Autodesk Inventor part; units mm, degrees
ref_plane "YZ Plane" through (0, 0, 0) normal (1, 0, 0) x (0, 1, 0)
ref_plane "XZ Plane" through (0, 0, 0) normal (0, 1, 0) x (-1, 0, 0)
ref_plane "XY Plane" through (0, 0, 0) normal (0, 0, 1) x (1, 0, 0)
sketch "Sketch1" plane through (0, 0, 0) normal (0, 0, 1) x (1, 0, 0)
  circle A0 centre (0, 0) radius 10
  dimension "d0" = 20
extrude "Extrusion1" add sketch "Sketch1" along normal blind 2
sketch "Sketch2" plane through (0, 0, 0) normal (0, 0, -1) x (-1, 0, 0)
  circle A0 centre (0, 0) radius 5.5
  circle A1 centre (0, 0) radius 3.55
  dimension "d3" = 11
  dimension "d6" = 7.1
extrude "Extrusion2" add sketch "Sketch2" against normal blind 30 contours A0 | A1
sketch "Sketch3" plane through (0, 0, 0) normal (0, 0, -1) x (-1, 0, 0)
  point P0 (0, 0)
sketch "Sketch4" plane through (0, 0, 0) normal (0, 0, -1) x (-1, 0, 0)
  point P0 (0, 0)
sketch "Sketch5" plane through (0, 0, 0) normal (0, 0, -1) x (-1, 0, 0)
  circle A0 centre (0, 0) radius 4
  dimension "d7" = 8
extrude "Extrusion3" cut sketch "Sketch5" against normal blind 30
sketch "Sketch6" plane through (0, 0, 2) normal (0, 0, 1) x (1, 0, 0)
  circle A0 centre (7, 2) radius 1
  circle A1 centre (7, -2) radius 1
  circle A2 centre (-7, 2) radius 1
  circle A3 centre (-7, -2) radius 1
  point P0 (0, 0)
  dimension "d16" = 2
  dimension "d17" = 7
  dimension "d18" = 2
  dimension "d19" = 2
  dimension "d20" = 7
  dimension "d21" = 2
  dimension "d53" = 2
  dimension "d54" = 7
  dimension "d55" = 2
  dimension "d56" = 2
  dimension "d57" = 7
  dimension "d58" = 2
extrude "Extrusion4" cut sketch "Sketch6" against normal blind 2
sketch "Sketch7" plane through (0, 0, 0) normal (0, 0, -1) x (-1, 0, 0)
  point P0 (0, 0)
sketch "Sketch8" plane through (0, 0, 0) normal (0, 0, -1) x (-1, 0, 0)
  circle A0 centre (-29.1938, 0) radius 12
  point P0 (0, 0)
  dimension "d24" = 24
extrude "Extrusion5" add sketch "Sketch8" against normal blind 2
sketch "Sketch9" plane through (29.1938, 0, 0) normal (0, 0, -1) x (-1, 0, 0)
  circle A0 centre (0, 0) radius 6
  point P0 (29.1938, 0)
  dimension "d27" = 12
extrude "Extrusion6" cut sketch "Sketch9" against normal blind 1
sketch "Sketch10" plane through (29.1938, 0, 0) normal (0, 0, -1) x (-1, 0, 0)
  point P0 (29.1938, 0)
  point P1 (0, 0)
sketch "Sketch11" plane through (29.1938, 0, 0) normal (0, 0, -1) x (-1, 0, 0)
  circle A0 centre (7.6938, 2) radius 1
  circle A1 centre (-8.3062, 2) radius 1
  circle A2 centre (-8.3062, -2) radius 1
  circle A3 centre (7.6938, -2) radius 1
  point P0 (29.1938, 0)
  dimension "d30" = 21.5
  dimension "d31" = 2
  dimension "d32" = 16
  dimension "d33" = 2
  dimension "d34" = 2
  dimension "d35" = 0
  dimension "d36" = 0
  dimension "d37" = 4
  dimension "d38" = 2
  dimension "d40" = 2
  dimension "d41" = 4
extrude "Extrusion7" cut sketch "Sketch11" against normal blind 2
sketch "Sketch12" plane through (29.1938, 0, 2) normal (0, 0, 1) x (1, 0, 0)
  circle A0 centre (0, 0) radius 4.55
  point P0 (-29.1938, 0)
  dimension "d44" = 9.1
extrude "Extrusion8" cut sketch "Sketch12" against normal blind 1
sketch "Sketch13" plane through (29.1938, 0, 0) normal (0, 0, -1) x (-1, 0, 0)
  line L0 (19.6938, 1) -> (11.6938, 1)
  line L1 (11.6938, 1) -> (11.6938, -1)
  line L2 (11.6938, -1) -> (19.6938, -1)
  line L3 (19.6938, -1) -> (19.6938, 1)
  point P0 (29.1938, 0)
  dimension "d47" = 8
  dimension "d48" = 2
  dimension "d49" = 1
  dimension "d50" = 9.5
extrude "Extrusion9" add sketch "Sketch13" against normal blind 1
sketch "Sketch14" plane through (29.1938, 0, 2) normal (0, 0, 1) x (1, 0, 0)
  point P0 (-29.1938, 0)
sketch "Sketch15" plane through (29.1938, 0, 2) normal (0, 0, 1) x (1, 0, 0)
  circle A0 centre (0, 0) radius 12
  point P0 (-29.1938, 0)
  dimension "d59" = 24
extrude "Extrusion10" add sketch "Sketch15" along normal blind 22
sketch "Sketch16" plane through (29.1938, 0, 24) normal (0, 0, 1) x (1, 0, 0)
  circle A0 centre (0, 0) radius 10.5
  point P0 (-29.1938, 0)
  dimension "d62" = 21
extrude "Extrusion11" cut sketch "Sketch16" against normal blind 23
properties part number "Bobbin01"
Could you check a few things on this model? Use its own coordinates, in mm. A direction names the side the tool comes from. Give positions to 0.01 mm unless a question says otherwise; leave off trailing zeros. Order: outer loops, then holes, each group sorted by start corner. A loop starts at its lowest first (then second) coordinate and runs counter-clockwise, first axis right, second up.
1. Suppose I cut it at A-A (x = 0). Write out the boundary of the cut face in (y, z).
Answers below:
outline: (-10, 0) - (-4, 0) - (-4, 30) - (-5.5, 30) - (-5.5, 2) - (-10, 2) - close; (4, 0) - (10, 0) - (10, 2) - (5.5, 2) - (5.5, 30) - (4, 30) - close
2. Suppose I cut it at B-B (y = 0). Write out the boundary of the cut face in (x, z), plus the area to 3 significant figures.
Answers below:
outline: (-10, 0) - (-4, 0) - (-4, 30) - (-5.5, 30) - (-5.5, 2) - (-10, 2) - close; (4, 0) - (23.19, 0) - (23.19, 1) - (18.69, 1) - (18.69, 24) - (17.19, 24) - (17.19, 1) - (10, 1) - (10, 2) - (5.5, 2) - (5.5, 30) - (4, 30) - close; (35.19, 0) - (41.19, 0) - (41.19, 24) - (39.69, 24) - (39.69, 1) - (35.19, 1) - close
area: 196 mm2
3. Thinking about a two-plate mould opening in Y: for faces 1 (the cylindrical face through (20.576, 1.617, 0.493)), 2 (the cylindrical face through (6.2, 1.4, 1)), 3 (the flat face through (15, 0, 0)), 4 (the flat face through (13.5, 1, 0.5)), which applies, +Y half, -Y half, draft (parallel to the pull), parting line (faces both ways), or undercut?
Answers below:
face 1: undercut
face 2: undercut
face 3: draft
face 4: +Y half
4. Suppose I cut it at D-D (x = 21.5). Write out the boundary of the cut face in (y, z).
Answers below:
outline: (-9.21, 0) - (-3, 0) - (-3, 1) - (-7.15, 1) - (-7.15, 24) - (-9.21, 24) - close; (-1, 0) - (1, 0) - (1, 1) - (-1, 1) - close; (3, 0) - (9.21, 0) - (9.21, 24) - (7.15, 24) - (7.15, 1) - (3, 1) - close
5. For pin 1 (1.5 mm diameter, centred on y = 1.5, z = 9, fed in from -X); pin 2 (6 mm diameter, centred on x = 33, z = 11, fed in from -Y); pin 3 (12 mm diameter, centred on x = 27.5, y = -5.5, fed in from +Z), each with a flat end and sliding along its axis, tell me the tip position at first contact or that it passes through.
Answers below:
pin 1: stops at x = -5.45
pin 2: stops at y = -11.97
pin 3: stops at z = 24
6. Which directions (+Z, -Z, +X, -X, +Y, -Y) give clear straight access to the entire face, cutting with the end or side of a thin tool? Please do faces 5 (the flat face through (4, -4, 2)), 6 (the flat face through (29, -11, 24)), 7 (the flat face through (14, 0, 1)).
Answers below:
face 5: +Z
face 6: +Z, +X, +Y, -Y
face 7: +Z, +Y, -Y
7. I need wall thicknesses on L1, parallel to Y at x = -7, z = 0.9; L2, parallel to Y at x = 0, z = 25.5; L3, parallel to Y at x = 29, z = 20.25. Which ranges of each line are inside material? Lowest first, please.
Answers below:
L1: y = -7.14 to -3, -1 to 1, 3 to 7.14
L2: y = -5.5 to -4, 4 to 5.5
L3: y = -12 to -10.5, 10.5 to 12
8. Suppose I cut it at C-C (z = 4.25). Write out the boundary of the cut face in (x, y).
Answers below:
outline: circle Ø11 at (0, 0); circle Ø24 at (29.19, 0); hole circle Ø8 at (0, 0); hole circle Ø21 at (29.19, 0)
